Part model, mm, in its own coordinate system. A direction names the side the tool comes from. Coordinates: 2 decimals unless noted, no trailing zeros. Loops run counter-clockwise (first coordinate to the right, second up) from the corner with the lowest first, then second, coordinate; pieces in that order, holes last. Notation, with made-up numbers: M 11.5,14 L 66.5,14 A11 cw 66.5,18 Z; hole C -0.75,87.5 d2. An arc over 180 degrees is marked long. Use a Markdown table: item, result. Add a question column.
1) Tool access for faces 1 (the cylindrical face through (2.3, -90.51, 0.99)), 2 (the cylindrical face through (20.72, 61.95, 1.01)): list every direction of +Z, -Z, +X, -X, +Y, -Y with a clear straight run to the whole face (end or side of a thin tool).
2) Pin check, flat tips, straight feed: pin 1 Ø0.6 at (y, z) = (-30.5, 1) entering from -X; pin 2 Ø0.6 at (x, z) = (4, 1) entering from -Y. Stop position of each tip, or through.
3) Band-saw the part on C-C (y = 139). List the corners of the cut face in (x, z).
4) Band-saw the part on B-B (z = 0.7). State how many separate pieces and enclosed holes the cut face has, plus the area to 3 significant figures.
5) Pull direction X, two halves, no side cores. Call faces 3 (the cylindrical face through (3.2, 230.535, 0.986)), 4 (the flat face through (20.64, 125.14, 0.99)), 5 (the cylindrical face through (-19.024, 79.978, 1.014)), 6 (the flat face through (-22.207, 196.699, 0.986)): released by +X, released by -X, zero draft, split by the parting line, or undercut.
6) Band-saw the part on A-A (y = 98). List the corners of the cut face in (x, z), plus the area to 3 significant figures.
7) Wall check: probe 1 along X at (y, z) = (172.5, 1.4); probe 2 along X at (y, z) = (38, 0.35); probe 3 along Y at (x, z) = (-7.5, 1.2) (1 decimal). Give the ranges that are in metal, low to high. Write a range as from..to.
from build123d import *

# Parameters (mm, degrees)
SKETCH_1_R      = 9.55
SKETCH_1_R_2    = 2.55
SKETCH_1_W      = 6.2
SKETCH_1_H      = 6.2
EXTRUDE_2_DEPTH = 2
FILLET_1_R      = 6
FILLET_2_R      = 14
FILLET_3_R      = 2


with BuildPart() as part:
    # 草图1 → 凸台-拉伸2 (new body)
    with BuildSketch(Plane.XY):
        with BuildLine():
            Line((-17.779440223, 210.011697354), (-26.761097666, 183.008415033))
            Line((-26.761097666, 183.008415033), (-30.283015797, 70.011697354))
            Line((-30.283015797, 70.011697354), (-26.761097666, -42.985020326))
            Line((-26.761097666, -42.985020326), (-17.779440223, -69.988302646))
            ThreePointArc((-17.779440223, -69.988302646), (2.748608262, -90.516351131), (23.276656746, -69.988302646))
            Line((23.276656746, -69.988302646), (32.258314189, -42.985020326))
            Line((32.258314189, -42.985020326), (35.78023232, 70.011697354))
            Line((35.78023232, 70.011697354), (32.258314189, 183.008415033))
            Line((32.258314189, 183.008415033), (23.276656746, 210.011697354))
            ThreePointArc((23.276656746, 210.011697354), (2.748608262, 230.539745838), (-17.779440223, 210.011697354))
        make_face()
        with Locations((2.748608262, 210.011697354)):
            Circle(SKETCH_1_R, mode=Mode.SUBTRACT)
        with Locations((-2.251391738, 165.011697354)):
            Circle(SKETCH_1_R_2, mode=Mode.SUBTRACT)
        with Locations((7.748608262, 165.011697354)):
            Circle(SKETCH_1_R_2, mode=Mode.SUBTRACT)
        with Locations((7.748608262, -24.988302646)):
            Circle(SKETCH_1_R_2, mode=Mode.SUBTRACT)
        with Locations((-2.251391738, -24.988302646)):
            Circle(SKETCH_1_R_2, mode=Mode.SUBTRACT)
        with Locations((2.748608262, -69.988302646)):
            Circle(SKETCH_1_R, mode=Mode.SUBTRACT)
        with Locations((-18.251391738, 152.961697354)):
            Rectangle(SKETCH_1_W, SKETCH_1_H, mode=Mode.SUBTRACT)
        with Locations((-18.251391738, 170.061697354)):
            Rectangle(SKETCH_1_W, SKETCH_1_H, mode=Mode.SUBTRACT)
        Polygon((26.399526511, 93.573959612), (-9.02733062, 147.961697354), (16.478190756, 147.961697354), align=None, mode=Mode.SUBTRACT)
        Polygon((-15.205972232, 139.125442928), (-24.505459679, 75.011697354), (26.556171202, 75.011697354), align=None, mode=Mode.SUBTRACT)
        with Locations((23.748608262, 152.961697354)):
            Rectangle(SKETCH_1_W, SKETCH_1_H, mode=Mode.SUBTRACT)
        with Locations((23.748608262, 170.061697354)):
            Rectangle(SKETCH_1_W, SKETCH_1_H, mode=Mode.SUBTRACT)
        with Locations((23.748608262, -30.038302646)):
            Rectangle(SKETCH_1_W, SKETCH_1_H, mode=Mode.SUBTRACT)
        with Locations((23.748608262, -12.938302646)):
            Rectangle(SKETCH_1_W, SKETCH_1_H, mode=Mode.SUBTRACT)
        with Locations((-18.251391738, -12.938302646)):
            Rectangle(SKETCH_1_W, SKETCH_1_H, mode=Mode.SUBTRACT)
        Polygon((26.556171202, 65.011697354), (-15.205972232, 0.897951779), (-24.505459679, 65.011697354), align=None, mode=Mode.SUBTRACT)
        Polygon((16.478190756, -7.938302646), (26.399526511, 46.449435095), (-9.02733062, -7.938302646), align=None, mode=Mode.SUBTRACT)
        with Locations((-18.251391738, -30.038302646)):
            Rectangle(SKETCH_1_W, SKETCH_1_H, mode=Mode.SUBTRACT)
    extrude(amount=EXTRUDE_2_DEPTH)

    # 圆角1
    fillet_1_edges = [part.edges().sort_by_distance(p)[0] for p in [
        (-15.205972232, 139.125442928, 1),
        (26.556171202, 75.011697354, 1),
        (26.556171202, 65.011697354, 1),
        (-15.205972232, 0.897951779, 1),
    ]]
    fillet(fillet_1_edges, radius=FILLET_1_R)

    # 圆角2
    fillet_2_edges = [part.edges().sort_by_distance(p)[0] for p in [
        (-24.505459679, 75.011697354, 1),
        (-24.505459679, 65.011697354, 1),
    ]]
    fillet(fillet_2_edges, radius=FILLET_2_R)

    # 圆角3
    fillet_3_edges = [part.edges().sort_by_distance(p)[0] for p in [
        (-9.02733062, -7.938302646, 1),
        (16.478190756, -7.938302646, 1),
        (26.399526511, 46.449435095, 1),
        (-9.02733062, 147.961697354, 1),
        (26.399526511, 93.573959612, 1),
        (16.478190756, 147.961697354, 1),
    ]]
    fillet(fillet_3_edges, radius=FILLET_3_R)


solid = part.part
Entries:
| question | item | result |
|---|---|---|
| 1 | face 1 | +Z, -Z, -Y |
| 1 | face 2 | +Z, -Z |
| 2 | pin 1 | x = -27.16 |
| 2 | pin 2 | y = -90.49 |
| 3 | outline | M -28.13,0 L -3.19,0 L -3.19,2 L -28.13,2 Z; M 18.11,0 L 33.63,0 L 33.63,2 L 18.11,2 Z |
| 4 | separate pieces | 1 |
| 4 | enclosed holes | 18 |
| 4 | area | 12,800 mm2 |
| 5 | face 3 | split by the parting line |
| 5 | face 4 | undercut |
| 5 | face 5 | undercut |
| 5 | face 6 | released by -X |
| 6 | outline | M -29.41,0 L -21.17,0 L -21.17,2 L -29.41,2 Z; M 11.58,0 L 34.91,0 L 34.91,2 L 11.58,2 Z |
| 6 | area | 63.1 mm2 |
| 7 | probe 1 | -27.09..-21.35, -15.15..20.65, 26.85..32.59 |
| 7 | probe 2 | -29.29..-20.59, 8.96..20.9, 24.39..34.78 |
| 7 | probe 3 | -87.8..13.1, 65..75, 126.9..227.8 |
